Here's the drawing with two shaded views (mm, measured from the low corner). I have some questions. A direction names the side the tool comes from. Coordinates: 2 decimals unless noted, no trailing zeros. Loops run counter-clockwise (first coordinate to the right, second up) from the corner with the lowest first, then second, coordinate; pieces in that order, holes last. Notation, with made-up numbers: (46, 12.5) -> (52, 12.5) arc R27 cw to (52, 42.5) -> close; hole circle Ø2 at (45.25, 74.5). An arc over 180 degrees is marked (long way). Answer as a JSON object with one key per item and string values. Group by question number.
1) I want a section at A-A (x = 11.5). Write out the boundary of the cut face in (y, z), then the cut area to 3 significant figures.
2) Which directions (+Z, -Z, +X, -X, +Y, -Y) give clear straight access to the entire face, cutting with the end or side of a thin tool? Please do the marked faces 4 and 5.
3) I want a section at B-B (z = 11.5). Write out the boundary of the cut face in (x, y), then the cut area to 3 significant figures.
4) I'm going to push flat-ended pins straight in: pin 1 (1.5 mm diameter, centred on x = 15.5, y = 3.5, fed in from -Z); pin 2 (1 mm diameter, centred on x = 14, y = 3.5, fed in from -Z); pin 3 (4 mm diameter, centred on x = 16.45, z = 6.55, fed in from +Y). Where does each tip first touch, or does it pass through?
5) I need wall thicknesses on probe 1 along Z at (x, y) = (15.75, 0.35) (1 decimal); probe 2 along Y at (x, z) = (7.75, 6); probe 3 along X at (y, z) = (0.7, 11.5). Which ranges of each line are inside material? Lowest first, please. Write a range as [from, to].
6) I want a section at C-C (y = 3.6). Write out the boundary of the cut face in (x, z).
7) If we mould it in two halves opening along Z, with no side actions, what happens to the marked faces 1, 2 and 3? For each: +Z half, -Z half, draft (parallel to the pull), parting line (faces both ways), or undercut.
8) I want a section at D-D (y = 1.2). Write out the boundary of the cut face in (x, z).
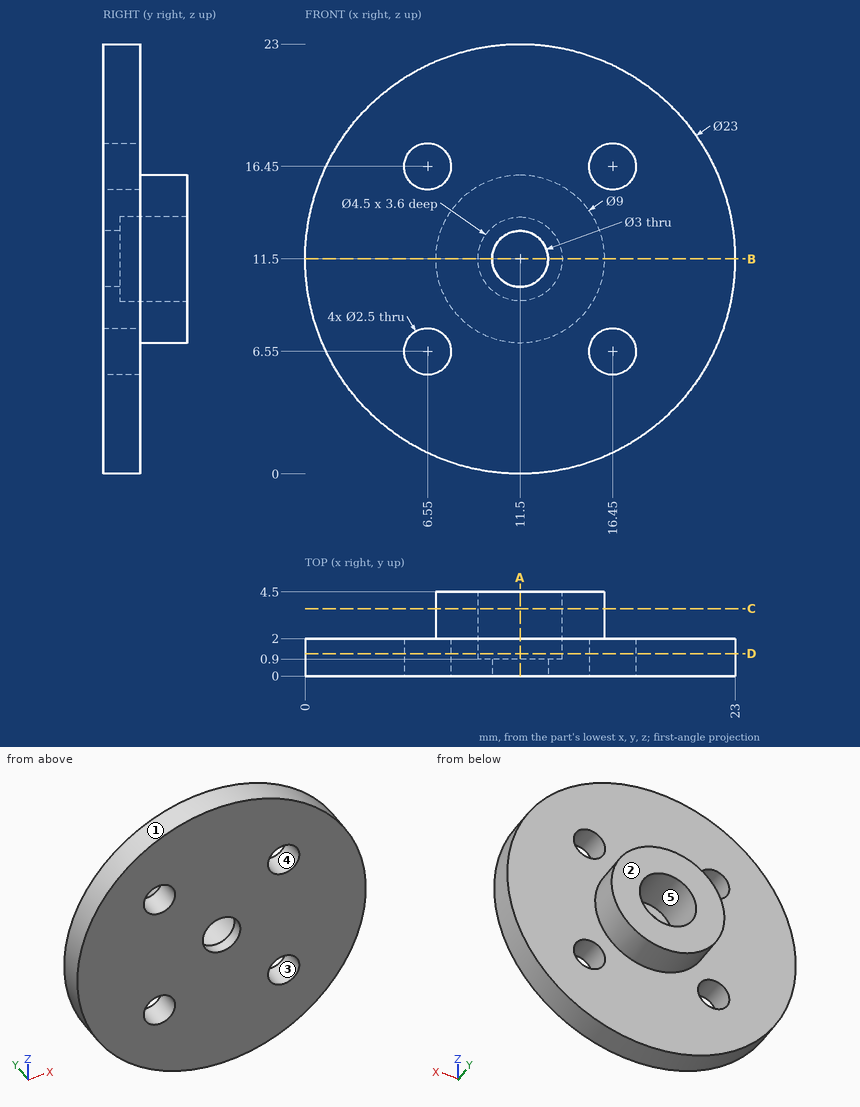
Determined:
{
 "1": {"outline": "(0, 0) -> (2, 0) -> (2, 7) -> (4.5, 7) -> (4.5, 9.25) -> (0.9, 9.25) -> (0.9, 10) -> (0, 10) -> close; (0, 13) -> (0.9, 13) -> (0.9, 13.75) -> (4.5, 13.75) -> (4.5, 16) -> (2, 16) -> (2, 23) -> (0, 23) -> close", "area": "49.6 mm^2"},
 "2": {"face 4": "+Y, -Y", "face 5": "+Y"},
 "3": {"outline": "(0, 0) -> (10, 0) -> (10, 0.9) -> (9.25, 0.9) -> (9.25, 4.5) -> (7, 4.5) -> (7, 2) -> (0, 2) -> close; (13, 0) -> (23, 0) -> (23, 2) -> (16, 2) -> (16, 4.5) -> (13.75, 4.5) -> (13.75, 0.9) -> (13, 0.9) -> close", "area": "49.6 mm^2"},
 "4": {"pin 1": "z = 8.39", "pin 2": "z = 7.47", "pin 3": "y = 2"},
 "5": {"probe 1": "[0.8, 5.5], [7.6, 15.4], [17.5, 22.2]", "probe 2": "[0, 2]", "probe 3": "[0, 10], [13, 23]"},
 "6": {"outline": "circle Ø9 at (11.5, 11.5); hole circle Ø4.5 at (11.5, 11.5)"},
 "7": {"face 1": "parting line", "face 2": "draft", "face 3": "undercut"},
 "8": {"outline": "circle Ø23 at (11.5, 11.5); hole circle Ø2.5 at (6.55, 6.55); hole circle Ø2.5 at (6.55, 16.45); hole circle Ø4.5 at (11.5, 11.5); hole circle Ø2.5 at (16.45, 6.55); hole circle Ø2.5 at (16.45, 16.45)"}
}
